```python
from build123d import *

# Parameters (mm, degrees)
SKETCH1_W           = 46
SKETCH1_H           = 36
BOSS_EXTRUDE1_DEPTH = 15
BOSS_EXTRUDE2_DEPTH = 3
SKETCH3_R           = 7.75
SKETCH3_R_2         = 9
CUT_EXTRUDE1_DEPTH  = 10
SKETCH4_W           = 5
SKETCH4_H           = 5
SKETCH4_R           = 1
BOSS_EXTRUDE3_DEPTH = 10
FILLET1_R           = 2.5
SKETCH6_R           = 1
CUT_EXTRUDE2_DEPTH  = 10
CHAMFER1_SIZE       = 2
FILLET2_R           = 2
SKETCH7_W           = 13
SKETCH7_H           = 4.5
CUT_EXTRUDE3_DEPTH  = 10
SKETCH8_W           = 9
SKETCH8_H           = 4
CUT_EXTRUDE4_DEPTH  = 10
SKETCH9_W           = 2
SKETCH9_H           = 4
CUT_EXTRUDE5_DEPTH  = 10


with BuildPart() as part:
    # Sketch1 → Boss-Extrude1 (new body)
    with BuildSketch(Plane.XY):
        Polygon((-15, -27.5), (-15, -20), (25, -20), (25, 20), (5, 20), (5, 27.5), (-25, 27.5), (-25, -27.5), align=None)
        Rectangle(SKETCH1_W, SKETCH1_H, mode=Mode.SUBTRACT)
    extrude(amount=BOSS_EXTRUDE1_DEPTH)

    # Sketch2 → Boss-Extrude2 (add)
    with BuildSketch(Plane.XY.offset(15)):
        Polygon((-25, 27.5), (-25, -27.5), (-15, -27.5), (-15, -20), (25, -20), (25, 20), (5, 20), (5, 27.5), align=None)
    extrude(amount=BOSS_EXTRUDE2_DEPTH)

    # Sketch3 → Cut-Extrude1 (cut)
    with BuildSketch(Plane.XY.offset(18)):
        with Locations((-10.25, 0)):
            Circle(SKETCH3_R)
        with Locations((12, 0)):
            Circle(SKETCH3_R_2)
    extrude(amount=-CUT_EXTRUDE1_DEPTH, mode=Mode.SUBTRACT)

    # Sketch4 → Boss-Extrude3 (add)
    # profile 1 of 4: a face of its own
    with BuildSketch(Plane(origin=(0, 0, 15), x_dir=(-1, 0, 0), z_dir=(0, 0, -1))):
        with Locations((20.5, -15.5)):
            Rectangle(SKETCH4_W, SKETCH4_H)
        with Locations((20.252039878, -15.196246514)):
            Circle(SKETCH4_R, mode=Mode.SUBTRACT)
    # profile 2 of 4: a face of its own
    with BuildSketch(Plane(origin=(0, 0, 15), x_dir=(-1, 0, 0), z_dir=(0, 0, -1))):
        with Locations((-3.747960122, -15.5)):
            Rectangle(SKETCH4_W, SKETCH4_H)
        with Locations((-3.747960122, -15.196246514)):
            Circle(SKETCH4_R, mode=Mode.SUBTRACT)
    # profile 3 of 4: a face of its own
    with BuildSketch(Plane(origin=(0, 0, 15), x_dir=(-1, 0, 0), z_dir=(0, 0, -1))):
        with Locations((-3.747960122, 15.5)):
            Rectangle(SKETCH4_W, SKETCH4_H)
        with Locations((-3.747960122, 15.203753486)):
            Circle(SKETCH4_R, mode=Mode.SUBTRACT)
    # profile 4 of 4: a face of its own
    with BuildSketch(Plane(origin=(0, 0, 15), x_dir=(-1, 0, 0), z_dir=(0, 0, -1))):
        with Locations((20.5, 15.5)):
            Rectangle(SKETCH4_W, SKETCH4_H)
        with Locations((20.252039878, 15.203753486)):
            Circle(SKETCH4_R, mode=Mode.SUBTRACT)
    extrude(amount=BOSS_EXTRUDE3_DEPTH)

    # Fillet1
    fillet1_edges = [part.edges().sort_by_distance(p)[0] for p in [
        (1.247960122, 13, 10),
        (6.247960122, 13, 10),
        (-18, 13, 10),
        (-18, -13, 10),
        (1.247960122, -13, 10),
        (6.247960122, -13, 10),
    ]]
    fillet(fillet1_edges, radius=FILLET1_R - 0.0001)  # a hair under: the kernel refuses the full size

    # Sketch6 → Cut-Extrude2 (cut)
    with BuildSketch(Plane(origin=(0, 0, -3), x_dir=(-1, 0, 0), z_dir=(0, 0, -1))):
        with Locations((0, 22.5)):
            Circle(SKETCH6_R)
        with Locations((20, 22.5)):
            Circle(SKETCH6_R)
        with Locations((20, -22.5)):
            Circle(SKETCH6_R)
    extrude(amount=-CUT_EXTRUDE2_DEPTH, mode=Mode.SUBTRACT)

    # Chamfer1
    chamfer1_edges = [part.edges().sort_by_distance(p)[0] for p in [
        (5, 27.5, 9),
        (5, 20, 9),
        (-15, -20, 9),
        (-15, -27.5, 9),
    ]]
    chamfer(chamfer1_edges, length=CHAMFER1_SIZE)

    # Fillet2
    fillet2_edges = [part.edges().sort_by_distance(p)[0] for p in [
        (-25, 27.5, 9),
        (25, 20, 9),
        (25, -20, 9),
        (-25, -27.5, 9),
    ]]
    fillet(fillet2_edges, radius=FILLET2_R)

    # Sketch7 → Cut-Extrude3 (cut)
    with BuildSketch(Plane.XZ.offset(-18)):
        with Locations((13.2, 2.25)):
            Rectangle(SKETCH7_W, SKETCH7_H)
    extrude(amount=-CUT_EXTRUDE3_DEPTH, mode=Mode.SUBTRACT)

    # Sketch8 → Cut-Extrude4 (cut)
    with BuildSketch(Plane(origin=(0, -18, 0), x_dir=(1, 0, 0), z_dir=(0, 1, 0))):
        Polygon((22.2, 0), (9.2, 0), (9.2, -4.5), (11.7, -4.5), (11.7, -9.5), (22.2, -9.5), align=None)
        with Locations((-3.8, -6.2)):
            Rectangle(SKETCH8_W, SKETCH8_H)
    extrude(amount=-CUT_EXTRUDE4_DEPTH, mode=Mode.SUBTRACT)

    # Sketch9 → Cut-Extrude5 (cut)
    with BuildSketch(Plane.ZY.offset(-23)):
        with Locations((5.65, 14.2)):
            Rectangle(SKETCH9_W, SKETCH9_H)
    extrude(amount=-CUT_EXTRUDE5_DEPTH, mode=Mode.SUBTRACT)


solid = part.part
```
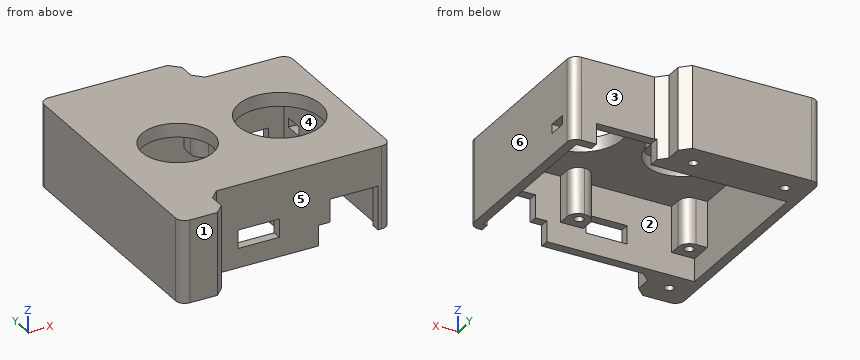
Geometry: final body of the model. Coordinates: model frame, mm. Face numbers are marked on the shaded views. A direction names the side the tool comes from. Coordinates: 2 decimals unless noted, no trailing zeros. Loops run counter-clockwise (first coordinate to the right, second up) from the corner with the lowest first, then second, coordinate; pieces in that order, holes last. Notation, with made-up numbers: (-25.75, -5.5) -> (-11.75, -5.5) arc R5 ccw to (-11.75, 1.5) -> close; hole circle Ø2 at (-9.5, -7). An arc over 180 degrees is marked (long way). Use a Markdown table: item, result. Add a question column.
(1) Section query D-D, the plane z = 15.75. Return loops of the section in (x, y), plus the area to 3 significant figures.
(2) Pin query (flat end, axial travel): pin 1 Ø0.6 at (x, y) = (3.5, -15) entering from -Z; pin 2 Ø2 at (y, z) = (-19, 5.5) entering from +X; pin 3 Ø4 at (y, z) = (-23, 11.5) entering from +X; pin 4 Ø0.6 at (y, z) = (-19, 8) entering from +X. Return the tip coordinate at first contact, or that it passes through.
(3) Mould query, pull axis X, two halves, no side actions, for the marked faces 4, 5 and 6. Classes: pulls with the +X half, pulls with the -X half, needs draft (parallel to the pull), parting line crosses it, or undercut.
(4) Section query C-C, the plane y = 0. Return loops of the section in (x, z).
(5) Section query B-B, the plane x = -10.25. Return loops of the section in (y, z).
(6) Section query A-A, the plane z = 1.5. State how many separate pieces and enclosed holes the cut face has, plus the area to 3 significant figures.
(7) Access query for the marked faces 1, 2 and 3. Directions: +Z, -Z, +X, -X, +Y, -Y. A direction counts if a zero-diameter tool reaches every point of the face in a straight line with its end or side. Return the directions, or none.
(8) Line query: line 1 along X through (y, z) = (12, 13.5); line 2 along Y through (x, z) = (12, 11.75); line 3 along Y through (x, z) = (0, 1.5). Output: solid intervals per line, ascending.
Answer:
| question | item | result |
|---|---|---|
| 1 | outline | (-25, -25.5) arc R2 ccw to (-23, -27.5) -> (-17, -27.5) -> (-15, -25.5) -> (-15, -22) -> (-13, -20) -> (23, -20) arc R2 ccw to (25, -18) -> (25, 18) arc R2 ccw to (23, 20) -> (7, 20) -> (5, 22) -> (5, 25.5) -> (3, 27.5) -> (-23, 27.5) arc R2 ccw to (-25, 25.5) -> close; hole circle Ø15.5 at (-10.25, 0); hole circle Ø18 at (12, 0) |
| 1 | area | 1,850 mm^2 |
| 2 | pin 1 | stops at z = 15 |
| 2 | pin 2 | stops at x = 25 |
| 2 | pin 3 | stops at x = -14 |
| 2 | pin 4 | stops at x = 24.87 |
| 3 | face 4 | undercut |
| 3 | face 5 | needs draft |
| 3 | face 6 | pulls with the +X half |
| 4 | outline | (-25, 0) -> (-23, 0) -> (-23, 15) -> (-18, 15) -> (-18, 18) -> (-25, 18) -> close; (-2.5, 15) -> (3, 15) -> (3, 18) -> (-2.5, 18) -> close; (21, 15) -> (23, 15) -> (23, 0) -> (25, 0) -> (25, 18) -> (21, 18) -> close |
| 5 | outline | (-20, 0) -> (-18, 0) -> (-18, 15) -> (-7.75, 15) -> (-7.75, 18) -> (-20, 18) -> close; (7.75, 15) -> (18, 15) -> (18, 0) -> (27.5, 0) -> (27.5, 18) -> (7.75, 18) -> close |
| 6 | separate pieces | 2 |
| 6 | enclosed holes | 3 |
| 6 | area | 579 mm^2 |
| 7 | face 1 | +Z, -Z, +X, -X, -Y |
| 7 | face 2 | -Z |
| 7 | face 3 | +Z, -Z, +X, +Y |
| 8 | line 1 | x = -25 to -23, 23 to 25 |
| 8 | line 2 | y = -20 to -18, 18 to 20 |
| 8 | line 3 | y = -20 to -18, 18 to 21.5, 23.5 to 27.5 |
